Geometry check sheet. Reference: the model listing, model coordinates, mm. A direction names the side the tool comes from. Round coordinates to 2 decimals unless told otherwise and drop trailing zeros. Loops run counter-clockwise (first coordinate to the right, second up) from the corner with the lowest first, then second, coordinate; pieces in that order, holes last. Notation, with made-up numbers: (42, -1) - (93, -1) arc R23 cw to (93, 13) - close; hole circle Ø6 at (-40, 79). An arc over 180 degrees is marked (long way). Write item = value, one per line.
```python
from build123d import *

# Parameters (mm, degrees)
SKETCH1_W           = 12.3
SKETCH1_H           = 45.6
SKETCH1_R           = 1
SKETCH1_W_2         = 6
SKETCH1_H_2         = 7
BOSS_EXTRUDE1_DEPTH = 3.5
FILLET1_R           = 6
FILLET2_R           = 1.5
SKETCH2_R           = 5.15
SKETCH2_R_2         = 3.5
BOSS_EXTRUDE2_DEPTH = 2.5


with BuildPart() as part:
    # Sketch1 → Boss-Extrude1 (new body)
    with BuildSketch(Plane.XY.offset(10)):
        with Locations((-295.077990014, 317.125181865)):
            Rectangle(SKETCH1_W, SKETCH1_H)
        with Locations((-290.97531395, 316.822329318)):
            Circle(SKETCH1_R, mode=Mode.SUBTRACT)
        with Locations((-299.053504652, 316.822329318)):
            Circle(SKETCH1_R, mode=Mode.SUBTRACT)
        with Locations((-294.951374343, 310.476860406)):
            Rectangle(SKETCH1_W_2, SKETCH1_H_2, mode=Mode.SUBTRACT)
        with Locations((-295.040754442, 323.502825528)):
            Rectangle(SKETCH1_W_2, SKETCH1_H_2, mode=Mode.SUBTRACT)
    extrude(amount=BOSS_EXTRUDE1_DEPTH)

    # Fillet1
    fillet1_edges = [part.edges().sort_by_distance(p)[0] for p in [
        (-301.227990014, 339.925181865, 11.75),
        (-288.927990014, 339.925181865, 11.75),
        (-288.927990014, 294.325181865, 11.75),
        (-301.227990014, 294.325181865, 11.75),
    ]]
    fillet(fillet1_edges, radius=FILLET1_R)

    # Fillet2
    fillet2_edges = [part.edges().sort_by_distance(p)[0] for p in [
        (-291.951374343, 306.976860406, 11.75),
        (-291.951374343, 313.976860406, 11.75),
        (-297.951374343, 313.976860406, 11.75),
        (-297.951374343, 306.976860406, 11.75),
        (-292.040754442, 320.002825528, 11.75),
        (-292.040754442, 327.002825528, 11.75),
        (-298.040754442, 327.002825528, 11.75),
        (-298.040754442, 320.002825528, 11.75),
    ]]
    fillet(fillet2_edges, radius=FILLET2_R)

    # Sketch2 → Boss-Extrude2 (add)
    # profile 1 of 2: a face of its own
    with BuildSketch(Plane.XY.offset(13.5)):
        with Locations((-295.031286372, 333.66110815)):
            Circle(SKETCH2_R)
        with Locations((-295.031286372, 333.66110815)):
            Circle(SKETCH2_R_2, mode=Mode.SUBTRACT)
    # profile 2 of 2: a face of its own
    with BuildSketch(Plane.XY.offset(13.5)):
        with Locations(Location((-295.031286372, 300.589255581, 0), (0, 0, 180))):
            Circle(SKETCH2_R)
        with Locations(Location((-295.031286372, 300.589255581, 0), (0, 0, 180))):
            Circle(SKETCH2_R_2, mode=Mode.SUBTRACT)
    extrude(amount=BOSS_EXTRUDE2_DEPTH)


solid = part.part
```
(1) Section check D-D (y = 308). Enter the section's corners in (x, z).
Answers follow:
outline = (-301.23, 10) - (-297.87, 10) - (-297.87, 13.5) - (-301.23, 13.5) - close; (-292.03, 10) - (-288.93, 10) - (-288.93, 13.5) - (-292.03, 13.5) - close
(2) Scan lines: L1, parallel to Y at x = -297, z = 11; L2, parallel to X at y = 323, z = 11.75; L3, parallel to Y at x = -296.5, z = 12.5. Record each from-to range of solid material in increasing order. Write a range as [from, to].
Answers follow:
L1 = [294.59, 307.08], [313.87, 320.07], [326.93, 339.66]
L2 = [-301.23, -298.04], [-292.04, -288.93]
L3 = [294.46, 306.98], [313.98, 320], [327, 339.79]
(3) Section check B-B (z = 11.25). Enter the section's corners in (x, y), then the cut area to 3 significant figures.
Answers follow:
outline = (-301.23, 300.33) arc R6 ccw to (-295.23, 294.33) - (-294.93, 294.33) arc R6 ccw to (-288.93, 300.33) - (-288.93, 333.93) arc R6 ccw to (-294.93, 339.93) - (-295.23, 339.93) arc R6 ccw to (-301.23, 333.93) - close; hole circle Ø2 at (-299.05, 316.82); hole (-298.04, 321.5) arc R1.5 ccw to (-296.54, 320) - (-293.54, 320) arc R1.5 ccw to (-292.04, 321.5) - (-292.04, 325.5) arc R1.5 ccw to (-293.54, 327) - (-296.54, 327) arc R1.5 ccw to (-298.04, 325.5) - close; hole (-297.95, 308.48) arc R1.5 ccw to (-296.45, 306.98) - (-293.45, 306.98) arc R1.5 ccw to (-291.95, 308.48) - (-291.95, 312.48) arc R1.5 ccw to (-293.45, 313.98) - (-296.45, 313.98) arc R1.5 ccw to (-297.95, 312.48) - close; hole circle Ø2 at (-290.98, 316.82)
area = 444 mm²
(4) Section check A-A (y = 323). Enter the section's corners in (x, z).
Answers follow:
outline = (-301.23, 10) - (-298.04, 10) - (-298.04, 13.5) - (-301.23, 13.5) - close; (-292.04, 10) - (-288.93, 10) - (-288.93, 13.5) - (-292.04, 13.5) - close
(5) Section check C-C (x = -292.5). Enter the section's corners in (y, z).
Answers follow:
outline = (294.84, 10) - (307.32, 10) - (307.32, 13.5) - (305.07, 13.5) - (305.07, 16) - (303.01, 16) - (303.01, 13.5) - (298.17, 13.5) - (298.17, 16) - (296.1, 16) - (296.1, 13.5) - (294.84, 13.5) - close; (313.64, 10) - (320.42, 10) - (320.42, 13.5) - (313.64, 13.5) - close; (326.58, 10) - (339.41, 10) - (339.41, 13.5) - (338.15, 13.5) - (338.15, 16) - (336.08, 16) - (336.08, 13.5) - (331.24, 13.5) - (331.24, 16) - (329.18, 16) - (329.18, 13.5) - (326.58, 13.5) - close
(6) Mould release check, pull along X, two halves, no side actions. Record for faces 1 (the cylindrical face through (-290.73, 338.21, 11.77)), 2 (the flat face through (-292.041, 323, 12)), 3 (the flat face through (-301.228, 317, 12)): pulls with the +X half, pulls with the -X half, needs draft (parallel to the pull), parting line crosses it, or undercut.
Answers follow:
face_1 = pulls with the +X half
face_2 = undercut
face_3 = pulls with the -X half
(7) Set-up check for faces 4 (the cylindrical face through (-299.52, 338.12, 11.77)), 5 (the flat face through (-295, 301, 13.5)), 6 (the cylindrical face through (-297.52, 313.53, 11.77)): record each of +Z, -Z, +X, -X, +Y, -Y from which the full face is reachable in a straight line by a thin tool's end or side.
Answers follow:
face_4 = +Z, -Z, -X, +Y
face_5 = +Z
face_6 = +Z, -Z
(8) Gauge pin test, flat ends, axial feed: pin 1 (1 mm diameter, centred on x = -293.5, y = 314.5, fed in from +Z); pin 2 (3 mm diameter, centred on x = -297.5, z = 11.5, fed in from -Y); pin 3 (1 mm diameter, centred on x = -290.5, z = 12, fed in from +Y). Record the tip position at first contact, or that the pin passes through.
Answers follow:
pin_1 = 13.5
pin_2 = 294.38
pin_3 = 338.46
